Here's how the part is built. I have some questions about the finished solid (model axes, mm). A direction names the side the tool comes from. Round coordinates to 2 decimals unless told otherwise and drop trailing zeros. Order: outer loops, then holes, each group sorted by start corner. A loop starts at its lowest first (then second) coordinate and runs counter-clockwise, first axis right, second up. Notation, with made-up numbers: (39, 2) -> (54, 2) arc R7 ccw to (54, 10) -> close; hole circle Ø11 at (-11.75, -17.75). An arc over 180 degrees is marked (long way). Answer in a Markdown table with one row per item.
```python
from build123d import *

# Parameters (mm, degrees)
SKETCH1_R           = 6.4135
SKETCH1_R_2         = 2.413
SKETCH1_R_3         = 12.7
SKETCH1_R_4         = 1.778
BOSS_EXTRUDE1_DEPTH = 6.35
FILLET1_R           = 5.08


with BuildPart() as part:
    # Sketch1 → Boss-Extrude1 (new body)
    with BuildSketch(Plane.XY):
        with BuildLine():
            Line((-19.05, 19.05), (265.43, 19.05))
            ThreePointArc((265.43, 19.05), (270.818153673, 21.281846327), (273.05, 26.67))
            Line((273.05, 26.67), (273.05, 36.83))
            Line((273.05, 36.83), (311.15, 36.83))
            Line((311.15, 36.83), (311.15, 3.81))
            ThreePointArc((311.15, 3.81), (304.454461018, -12.354461018), (288.29, -19.05))
            Line((288.29, -19.05), (286.189260549, -19.05))
            Line((286.189260549, -19.05), (-19.05, -19.05))
            Line((-19.05, -19.05), (-19.05, 19.05))
        make_face()
        Circle(SKETCH1_R, mode=Mode.SUBTRACT)
        with Locations((0, 11.43)):
            Circle(SKETCH1_R_2, mode=Mode.SUBTRACT)
        with Locations((11.43, 0)):
            Circle(SKETCH1_R_2, mode=Mode.SUBTRACT)
        with Locations((0, -11.43)):
            Circle(SKETCH1_R_2, mode=Mode.SUBTRACT)
        with Locations((-11.43, 0)):
            Circle(SKETCH1_R_2, mode=Mode.SUBTRACT)
        with Locations((292.1, 20.066)):
            Circle(SKETCH1_R_3, mode=Mode.SUBTRACT)
        with Locations((278.638, 33.544763148)):
            Circle(SKETCH1_R_4, mode=Mode.SUBTRACT)
        with Locations((305.562, 33.544763148)):
            Circle(SKETCH1_R_4, mode=Mode.SUBTRACT)
        with Locations((305.562, 6.587236852)):
            Circle(SKETCH1_R_4, mode=Mode.SUBTRACT)
        with Locations((278.638, 6.587236852)):
            Circle(SKETCH1_R_4, mode=Mode.SUBTRACT)
    extrude(amount=BOSS_EXTRUDE1_DEPTH)

    # Fillet1
    fillet1_edges = [part.edges().sort_by_distance(p)[0] for p in [
        (311.15, 36.83, 3.175),
    ]]
    fillet(fillet1_edges, radius=FILLET1_R)


solid = part.part
```
1. Please list where these lines run through material, in increasing order: line 1 along Y through (x, z) = (0, 5); line 2 along X through (y, z) = (7, 0.75); line 3 along Y through (x, z) = (11.43, 1.75).
Numbers:
| item | result |
|---|---|
| line 1 | y = -19.05 to -13.84, -9.02 to -6.41, 6.41 to 9.02, 13.84 to 19.05 |
| line 2 | x = -19.05 to 276.91, 280.37 to 303.83, 307.29 to 311.15 |
| line 3 | y = -19.05 to -2.41, 2.41 to 19.05 |
2. For pin 1 Ø6.5 at (x, y) = (0, 11.43) entering from +Z; pin 2 Ø10.5 at (x, y) = (0, 0) entering from -Z, each with a flat end and sliding along its axis, tell me the tip position at first contact or that it passes through.
Numbers:
| item | result |
|---|---|
| pin 1 | stops at z = 6.35 |
| pin 2 | passes through |
3. Suppose I cut it at B-B on x = 224.5. Write out the boundary of the cut face in (y, z).
Numbers:
| item | result |
|---|---|
| outline | (-19.05, 0) -> (19.05, 0) -> (19.05, 6.35) -> (-19.05, 6.35) -> close |
4. For faces 1 (the face through (304.214, 23.881, 3.131)), 2 (the face through (121, 19.05, 3)), which set-ups out of +Z, -Z, +X, -X, +Y, -Y let a thin tool reach every point of the face, with its end or its side?
Numbers:
| item | result |
|---|---|
| face 1 | +Z, -Z |
| face 2 | +Z, -Z, -X, +Y |
5. Suppose I cut it at A-A on z = 2. State how many separate pieces and enclosed holes the cut face has, then the cut area to 3 significant figures.
Numbers:
| item | result |
|---|---|
| separate pieces | 1 |
| enclosed holes | 10 |
| area | 12,400 mm2 |
6. We'd pull the mould along X, two halves only. Please class faces 3 (the face through (273.05, 32, 3)), 4 (the face through (304.631, -12.176, 3.131)), 5 (the face through (6.117, 1.926, 3.131)), 6 (the face through (148, 3, 0)): released by +X, released by -X, zero draft, split by the parting line, or undercut.
Numbers:
| item | result |
|---|---|
| face 3 | released by -X |
| face 4 | released by +X |
| face 5 | undercut |
| face 6 | zero draft |
